The model under review builds one solid part; all positions refer to its coordinate system, in mm. A direction names the side the tool comes from. Coordinates: 2 decimals unless noted, no trailing zeros. Loops run counter-clockwise (first coordinate to the right, second up) from the corner with the lowest first, then second, coordinate; pieces in that order, holes last. Notation, with made-up numbers: M 60.25,33 L 116.25,33 A20 ccw 116.25,54 Z; hole C 10.5,-30 d11. An arc over 180 degrees is marked long. Return JSON: item names as keys, results as strings.
```python
from build123d import *

# Parameters (mm, degrees)
SKETCH1_W         = 48.34
SKETCH1_H         = 18
EXTRUDE_3_8_DEPTH = 9.63
SKETCH2_R         = 1.75
M4_DRILL_DEPTH    = 8
M4_DRILL2_START   = -8
SKETCH3_R         = 1.75
M4_DRILL2_DEPTH   = 8
SKETCH5_R         = 2.2
M5_DRILL_DEPTH    = 9.63
FILLET1_R         = 4


with BuildPart() as part:
    # Sketch1 → 3/8 (new body)
    with BuildSketch(Plane.XY):
        Rectangle(SKETCH1_W, SKETCH1_H)
    extrude(amount=EXTRUDE_3_8_DEPTH)

    # Sketch2 → M4_DRILL (cut)
    with BuildSketch(Plane.ZY.offset(24.17)):
        with Locations((4.815, 5)):
            Circle(SKETCH2_R)
        with Locations(Location((4.815, -5, 0), (0, 0, 180))):
            Circle(SKETCH2_R)
    extrude(amount=-M4_DRILL_DEPTH, mode=Mode.SUBTRACT)

    # Sketch3 → M4_DRILL2 (cut)
    with BuildSketch(Plane(origin=(24.17, 0, 0), x_dir=(0, 0, -1), z_dir=(1, 0, 0)).offset(M4_DRILL2_START)):
        with Locations((-4.815, -5)):
            Circle(SKETCH3_R)
        with Locations(Location((-4.815, 5, 0), (0, 0, 180))):
            Circle(SKETCH3_R)
    extrude(amount=M4_DRILL2_DEPTH, mode=Mode.SUBTRACT)

    # Sketch5 → M5_DRILL (cut)
    with BuildSketch(Plane(origin=(0, 0, 0), x_dir=(-1, 0, 0), z_dir=(0, 0, -1))):
        Circle(SKETCH5_R)
    extrude(amount=-M5_DRILL_DEPTH, mode=Mode.SUBTRACT)

    # Fillet1
    fillet1_edges = [part.edges().sort_by_distance(p)[0] for p in [
        (0, -9, 9.63),
        (0, -9, 0),
        (0, 9, 0),
        (0, 9, 9.63),
    ]]
    fillet(fillet1_edges, radius=FILLET1_R)


solid = part.part
```
1. Insertion check: pin 1 Ø4 at (y, z) = (5, 5) entering from -X; pin 2 Ø1.8 at (y, z) = (-5, 5.5) entering from -X; pin 3 Ø1.8 at (y, z) = (-5, 5) entering from +X; pin 4 Ø3.5 at (x, y) = (0, 0) entering from -Z. Each pin has a flat end and moves straight along its axis. Give the tip position at first contact, or say it passes through.
Check values:
{"pin 1": "x = -24.17", "pin 2": "x = -16.17", "pin 3": "x = 16.17", "pin 4": "through"}
2. Add section A-A on y = 0. Give the boundary of the cut face in (x, z).
Check values:
{"outline": "M -24.17,0 L -2.2,0 L -2.2,9.63 L -24.17,9.63 Z; M 2.2,0 L 24.17,0 L 24.17,9.63 L 2.2,9.63 Z"}
3. Machinability: for faces 1 (the face through (16.17, -5, 5)), 2 (the face through (-20.226, -3.935, 6.204)), 3 (the face through (24.17, 0, 5)), which of the approach directions +Z, -Z, +X, -X, +Y, -Y give a long, thin tool a straight path to every point of the face, cutting with its end or side? Answer none if there is none.
Check values:
{"face 1": "+X", "face 2": "-X", "face 3": "+Z, -Z, +X, +Y, -Y"}
4. Add section B-B on x = 0. Give the boundary of the cut face in (y, z).
Check values:
{"outline": "M -9,4 A4 ccw -5,0 L -2.2,0 L -2.2,9.63 L -5,9.63 A4 ccw -9,5.63 Z; M 2.2,0 L 5,0 A4 ccw 9,4 L 9,5.63 A4 ccw 5,9.63 L 2.2,9.63 Z"}
5. To check wall thickness, follow line 1 (Y direction, x = 1, z = 1.25); line 2 (X direction, y = 1, z = 8.25); line 3 (Y direction, x = 0.5, z = 5.25). State the ranges of each line that lie inside material, in increasing order.
Check values:
{"line 1": "-7.9 to -1.96, 1.96 to 7.9", "line 2": "-24.17 to -1.96, 1.96 to 24.17", "line 3": "-9 to -2.14, 2.14 to 9"}
6. Add section D-D on z = 8. Give the boundary of the cut face in (x, y), plus the area to 3 significant figures.
Check values:
{"outline": "M -24.17,-8.22 L 24.17,-8.22 L 24.17,8.22 L -24.17,8.22 Z; hole C 0,0 d4.4", "area": "780 mm²"}
7. Add section C-C on x = -8.5. Give the boundary of the cut face in (y, z), plus the area to 3 significant figures.
Check values:
{"outline": "M -9,4 A4 ccw -5,0 L 5,0 A4 ccw 9,4 L 9,5.63 A4 ccw 5,9.63 L -5,9.63 A4 ccw -9,5.63 Z", "area": "160 mm²"}
8. The part is to be moulded in two halves that separate along X. For faces 4 (the face through (0, 3, 9.63)), 5 (the face through (-2.1, 0.66, 4.75)), 6 (the face through (-24.17, 0, 5)), say which applies: released by +X, released by -X, zero draft, split by the parting line, or undercut.
Check values:
{"face 4": "zero draft", "face 5": "undercut", "face 6": "released by -X"}
